```python
from build123d import *

# Parameters (mm, degrees)
SKETCH_1_R          = 22.5
EXTRUDE_1_DEPTH     = 2.5
SKETCH_4_R          = 7.5
EXTRUDE_2_DEPTH     = 4
SKETCH_5_R          = 7.5
SKETCH_5_R_2        = 3.55
EXTRUDE_3_DEPTH     = 9
SKETCH_6_R          = 1.8
CUT_EXTRUDE_2_DEPTH = 6
FILLET_1_R          = 0.5
CUT_EXTRUDE_3_DEPTH = 34.068111528
SKETCH_8_R          = 7.500275011
SKETCH_8_R_2        = 5.5
CUT_EXTRUDE_4_DEPTH = 13


with BuildPart() as part:
    # 草图1 → 凸台-拉伸1 (new body)
    with BuildSketch(Plane.XY):
        Circle(SKETCH_1_R)
    extrude(amount=EXTRUDE_1_DEPTH)

    # 草图4 → 凸台-拉伸2 (add)
    with BuildSketch(Plane(origin=(0, 0, 0), x_dir=(-1, 0, 0), z_dir=(0, 0, -1))):
        Circle(SKETCH_4_R)
    extrude(amount=EXTRUDE_2_DEPTH)

    # 草图5 → 凸台-拉伸3 (add)
    # profile 1 of 3: a face of its own
    with BuildSketch(Plane(origin=(0, 0, -4), x_dir=(-1, 0, 0), z_dir=(0, 0, -1))):
        with Locations(Location((0, 0, 0), (0, 0, 239.61601222))):
            Circle(SKETCH_5_R)
        with Locations((-0.000237242, 0.000139094)):
            Circle(SKETCH_5_R_2, mode=Mode.SUBTRACT)
    # profile 2 of 3: a face of its own
    with BuildSketch(Plane(origin=(0, 0, -4), x_dir=(-1, 0, 0), z_dir=(0, 0, -1))):
        with BuildLine():
            ThreePointArc((-0.000237242, -3.549860906), (-1.803359534, -2.802983198), (-2.550237242, -0.999860906))
            Line((-2.550237242, -0.999860906), (-2.550237242, 1.000139094))
            ThreePointArc((-2.550237242, 1.000139094), (-1.803359534, 2.803261386), (-0.000237242, 3.550139094))
            ThreePointArc((-0.000237242, 3.550139094), (-3.550237242, 0.000139094), (-0.000237242, -3.549860906))
        make_face()
    # profile 3 of 3: a face of its own
    with BuildSketch(Plane(origin=(0, 0, -4), x_dir=(-1, 0, 0), z_dir=(0, 0, -1))):
        with BuildLine():
            ThreePointArc((2.549762758, -0.999860906), (1.80288505, -2.802983198), (-0.000237242, -3.549860906))
            ThreePointArc((-0.000237242, -3.549860906), (2.509991831, -2.510089979), (3.549762758, 0.000139094))
            ThreePointArc((3.549762758, 0.000139094), (2.509991831, 2.510368167), (-0.000237242, 3.550139094))
            ThreePointArc((-0.000237242, 3.550139094), (1.80288505, 2.803261386), (2.549762758, 1.000139094))
            Line((2.549762758, 1.000139094), (2.549762758, -0.999860906))
        make_face()
    extrude(amount=EXTRUDE_3_DEPTH)

    # 草图6 → 切除-拉伸2 (cut)
    with BuildSketch(Plane.XY.offset(2.5)):
        with Locations((0, 11)):
            Circle(SKETCH_6_R)
        with Locations((-8.838834765, 8.838834765)):
            Circle(SKETCH_6_R)
        with Locations((8.838834765, 8.838834765)):
            Circle(SKETCH_6_R)
        with Locations((8.838834765, -8.838834765)):
            Circle(SKETCH_6_R)
        with Locations((-8.838834765, -8.838834765)):
            Circle(SKETCH_6_R)
        with Locations((11, 0)):
            Circle(SKETCH_6_R)
        with Locations((0, -11)):
            Circle(SKETCH_6_R)
        with Locations((-11, 0)):
            Circle(SKETCH_6_R)
    extrude(amount=-CUT_EXTRUDE_2_DEPTH, mode=Mode.SUBTRACT)

    # 圆角1
    fillet_1_edges = [part.edges().sort_by_distance(p)[0] for p in [
        (0.000237242, -3.549860906, -13),
        (0.000237242, 3.550139094, -13),
        (-2.549762758, 0.000139094, -13),
        (2.550237242, 0.000139094, -13),
    ]]
    fillet(fillet_1_edges, radius=FILLET_1_R)

    # 草图7 → 切除-拉伸3 (cut, through all)
    with BuildSketch(Plane(origin=(0, 0, -4), x_dir=(-1, 0, 0), z_dir=(0, 0, -1))):
        with BuildLine():
            Line((-2.550237242, 1.000139094), (-2.550237242, -0.999860906))
            ThreePointArc((-2.550237242, -0.999860906), (-0.000237242, -3.549860906), (2.549762758, -0.999860906))
            Line((2.549762758, -0.999860906), (2.549762758, 1.000139094))
            ThreePointArc((2.549762758, 1.000139094), (-0.000237242, 3.550139094), (-2.550237242, 1.000139094))
        make_face()
    extrude(amount=-CUT_EXTRUDE_3_DEPTH, mode=Mode.SUBTRACT)

    # 草图8 → 切除-拉伸4 (cut)
    with BuildSketch(Plane(origin=(0, 0, -13), x_dir=(-1, 0, 0), z_dir=(0, 0, -1))):
        Circle(SKETCH_8_R)
        Circle(SKETCH_8_R_2, mode=Mode.SUBTRACT)
    extrude(amount=-CUT_EXTRUDE_4_DEPTH, mode=Mode.SUBTRACT)


solid = part.part
```
The listing builds one solid part. Answer for the finished solid, in the listing's coordinates (mm). A direction names the side the tool comes from. Coordinates: 2 decimals unless noted, no trailing zeros. Write each loop counter-clockwise with the first axis right and the second up, starting at its lowest first coordinate (ties: lowest second). Pieces come first, ordered by that corner, then holes.
Q1. Section B-B, the plane y = 0 is taken. Write down the section's boundary in (x, z).
Returned:
outline: (-22.5, 0) - (-12.8, 0) - (-12.8, 2.5) - (-22.5, 2.5) - close; (-9.2, 0) - (-5.5, 0) - (-5.5, -13) - (-3.05, -13) arc R0.5 ccw to (-2.55, -12.5) - (-2.55, 2.5) - (-9.2, 2.5) - close; (2.55, -12.5) arc R0.5 ccw to (3.05, -13) - (5.5, -13) - (5.5, 0) - (9.2, 0) - (9.2, 2.5) - (2.55, 2.5) - close; (12.8, 0) - (22.5, 0) - (22.5, 2.5) - (12.8, 2.5) - close
Q2. Section D-D, the plane y = 15 is taken. Write down the section's boundary in (x, z), then the cut area to 3 significant figures.
Returned:
outline: (-16.77, 0) - (16.77, 0) - (16.77, 2.5) - (-16.77, 2.5) - close
area: 83.9 mm2
Q3. The mould has two halves that part along Y. Classify faces 1 (the flat face through (3.24, -0.84, -13)), 2 (the cylindrical face through (-10.27, -9.93, 1.27)), 3 (the cylindrical face through (1.19, -5.37, -6.59)), 4 (the cylindrical face through (0.831, 9.403, 1.268)): released by +Y, released by -Y, zero draft, split by the parting line, or undercut.
Returned:
face 1: zero draft
face 2: undercut
face 3: split by the parting line
face 4: undercut
Q4. Which of the six approach directions +Z, -Z, +X, -X, +Y, -Y give full straight-line access (tool end or side, diameter ignored) to faces 5 (the flat face through (-2.55, 0, -5)), 6 (the flat face through (-5, -5, 0)), 7 (the flat face through (0, -5, 2.5))?
Returned:
face 5: +Z, -Z
face 6: -Z
face 7: +Z, +X, -X, +Y, -Y
Q5. Section C-C, the plane x = 4.5 is taken. Write down the section's boundary in (y, z), then the cut area to 3 significant figures.
Returned:
outline: (-22.05, 0) - (-3.16, 0) - (-3.16, -13) - (3.16, -13) - (3.16, 0) - (22.05, 0) - (22.05, 2.5) - (-22.05, 2.5) - close
area: 192 mm2
Q6. Section A-A, the plane z = -11.25 is taken. Write down the section's boundary in (x, y).
Returned:
outline: circle Ø11 at (0, 0); hole (-2.55, -1) arc R2.55 ccw to (2.55, -1) - (2.55, 1) arc R2.55 ccw to (-2.55, 1) - close
Q7. Given P1, Ø2, axis at y = 0, z = -2.5, coming from the -X side; P2, Ø10, axis at x = -14.5, y = -4, coming from the -Z side; P3, Ø2, axis at x = -11, y = 0, coming from the -Z side; P4, Ø2, axis at y = 6, z = -4, coming from the -X side, each flat-ended and moving along its own axis, determine where each tip first touches the part or whether it passes through.
Returned:
P1: stops at x = -5.5
P2: stops at z = 0
P3: passes through
P4: stops at x = -2.29
Q8. Find the intervals of material crossed by line 1 along Y through (x, z) = (0, 2.05); line 2 along Y through (x, z) = (9, 1.5); line 3 along Z through (x, y) = (-7.5, -12), in increasing order.
Returned:
line 1: y = -22.5 to -12.8, -9.2 to -3.55, 3.55 to 9.2, 12.8 to 22.5
line 2: y = -20.62 to -10.63, -7.05 to 7.05, 10.63 to 20.62
line 3: z = 0 to 2.5
